Source: CAD feature listing. Evaluate the final solid. Frame: model axes, mm. Face numbers are marked on the shaded views. A direction names the side the tool comes from. Round coordinates to 2 decimals unless told otherwise and drop trailing zeros. Write each loop counter-clockwise with the first axis right and the second up, starting at its lowest first coordinate (ties: lowest second). Pieces come first, ordered by that corner, then holes. Notation, with made-up numbers: (-32.5, -13.5) - (24.5, -13.5) arc R13 ccw to (24.5, 10.5) - close; hole circle Ø1 at (42.25, -34). An arc over 180 degrees is marked (long way). Write item = value, one per line. Start each with the question number.
```python
from build123d import *

# Parameters (mm, degrees)
SKETCH_1_W          = 26
SKETCH_1_H          = 18
EXTRUDE_1_DEPTH     = 3
SKETCH_2_W          = 3
SKETCH_2_H          = 18
EXTRUDE_2_DEPTH     = 20
SKETCH_3_W          = 3
SKETCH_3_H          = 18
EXTRUDE_3_DEPTH     = 18
SKETCH_4_R          = 1.5
CUT_EXTRUDE_1_DEPTH = 36.860842154
FILLET_1_R          = 3
SKETCH_5_R          = 5.5
CUT_EXTRUDE_2_DEPTH = 36.860842154
FILLET_2_R          = 3


with BuildPart() as part:
    # 草图1 → 凸台-拉伸1 (new body)
    with BuildSketch(Plane(origin=(0, 0, 0), x_dir=(1, 0, 0), z_dir=(0, 1, 0))):
        Rectangle(SKETCH_1_W, SKETCH_1_H)
    extrude(amount=EXTRUDE_1_DEPTH)

    # 草图2 → 凸台-拉伸2 (add)
    with BuildSketch(Plane(origin=(0, 3, 0), x_dir=(1, 0, 0), z_dir=(0, 1, 0))):
        with Locations((-11.5, 0)):
            Rectangle(SKETCH_2_W, SKETCH_2_H)
        with Locations((11.5, 0)):
            Rectangle(SKETCH_2_W, SKETCH_2_H)
    extrude(amount=EXTRUDE_2_DEPTH)

    # 草图3 → 凸台-拉伸3 (add)
    with BuildSketch(Plane.XZ):
        with Locations((-7.5, 0)):
            Rectangle(SKETCH_3_W, SKETCH_3_H)
        with Locations((7.5, 0)):
            Rectangle(SKETCH_3_W, SKETCH_3_H)
    extrude(amount=EXTRUDE_3_DEPTH)

    # 草图4 → 切除-拉伸1 (cut, through all)
    with BuildSketch(Plane.ZY.offset(13)):
        with Locations((-6, 20)):
            Circle(SKETCH_4_R)
        with Locations(Location((6, 20, 0), (0, 0, 180))):
            Circle(SKETCH_4_R)
        with Locations((6, 6)):
            Circle(SKETCH_4_R)
        with Locations(Location((-6, 6, 0), (0, 0, 180))):
            Circle(SKETCH_4_R)
    extrude(amount=-CUT_EXTRUDE_1_DEPTH, mode=Mode.SUBTRACT)

    # 圆角1
    fillet_1_edges = [part.edges().sort_by_distance(p)[0] for p in [
        (-11.5, 23, 9),
        (-11.5, 23, -9),
        (11.5, 23, -9),
        (11.5, 23, 9),
    ]]
    fillet(fillet_1_edges, radius=FILLET_1_R)

    # 草图5 → 切除-拉伸2 (cut, through all)
    with BuildSketch(Plane.ZY.offset(13)):
        with Locations((0, -9)):
            Circle(SKETCH_5_R)
    extrude(amount=-CUT_EXTRUDE_2_DEPTH, mode=Mode.SUBTRACT)

    # 圆角2
    fillet_2_edges = [part.edges().sort_by_distance(p)[0] for p in [
        (-7.5, -18, -9),
        (-7.5, -18, 9),
        (7.5, -18, 9),
        (7.5, -18, -9),
    ]]
    fillet(fillet_2_edges, radius=FILLET_2_R)


solid = part.part
```
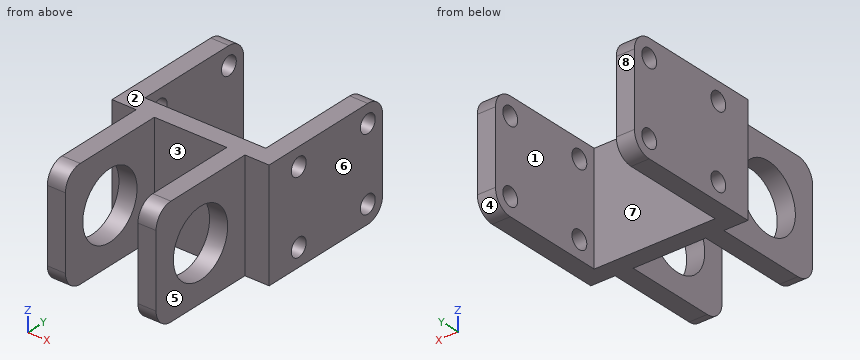
(1) Contact query for flat-ended pins moving along their axis: P1, Ø1.2, axis at x = -11, z = 3, coming from the -Y side; P2, Ø8, axis at y = -8, z = 5.5, coming from the +X side; P3, Ø5, axis at x = 1, z = -2.5, coming from the +Y side. Output: stop coordinate, or through.
(2) Section C-C (x = -8.5). Return the cut outline in (y, z).
(3) Section D-D (y = -9). Return the cut outline in (x, z), plus the area to 3 significant figures.
(4) Pull-direction query (X, two-part tool) for the marked faces 6, 7 and 8; classes: +X half, -X half, draft (parallel to the pull), parting line (faces both ways), or undercut.
(5) Section A-A (z = 0). Return the cut outline in (x, y), plus the area to 3 significant figures.
(6) Ray query, L1, parallel to Y at x = 11.3, z = -6; L2, parallel to Y at x = -8.05, z = 0; L3, parallel to X at y = -5.5, z = -6.25. Return the intervals inside material, ascending. Write a range as from..to.
(7) Reachability of the marked faces 1, 2, 3, 4 and 5 from +Z, -Z, +X, -X, +Y, -Y: full face, straight path, thin tool, end or side. Return the list, or none.
(8) Section B-B (y = -2). Return the cut outline in (x, z).
Solution:
q1.P1 = 0
q1.P2 = 9
q1.P3 = 3
q2.outline = (-18, -6) arc R3 ccw to (-15, -9) - (3, -9) - (3, 9) - (-15, 9) arc R3 ccw to (-18, 6) - close; hole circle Ø11 at (-9, 0)
q3.outline = (-9, -9) - (-6, -9) - (-6, -5.5) - (-9, -5.5) - close; (-9, 5.5) - (-6, 5.5) - (-6, 9) - (-9, 9) - close; (6, -9) - (9, -9) - (9, -5.5) - (6, -5.5) - close; (6, 5.5) - (9, 5.5) - (9, 9) - (6, 9) - close
q3.area = 42.0 mm^2
q4.face_6 = +X half
q4.face_7 = undercut
q4.face_8 = draft
q5.outline = (-13, 0) - (-9, 0) - (-9, -3.5) - (-6, -3.5) - (-6, 0) - (6, 0) - (6, -3.5) - (9, -3.5) - (9, 0) - (13, 0) - (13, 23) - (10, 23) - (10, 3) - (-10, 3) - (-10, 23) - (-13, 23) - close; (-9, -18) - (-6, -18) - (-6, -14.5) - (-9, -14.5) - close; (6, -18) - (9, -18) - (9, -14.5) - (6, -14.5) - close
q5.area = 240 mm^2
q6.L1 = 0..4.5, 7.5..18.5, 21.5..23
q6.L2 = -18..-14.5, -3.5..3
q6.L3 = -9..-6, 6..9
q7.face_1 = +Z, -Z, +Y
q7.face_2 = +Z, +X, -X, +Y, -Y
q7.face_3 = +Z, -Z, -Y
q7.face_4 = -Z, +X, -X, +Y
q7.face_5 = +Z, -Z, +X, -Y
q8.outline = (-9, -9) - (-6, -9) - (-6, 9) - (-9, 9) - close; (6, -9) - (9, -9) - (9, 9) - (6, 9) - close
